from build123d import *

# Parameters (mm, degrees)
SKETCH1_W               = 127
SKETCH1_H               = 127
BOSS_EXTRUDE1_DEPTH     = 6.35
BOSS_EXTRUDE2_DEPTH     = 6.35
BOSS_EXTRUDE3_DEPTH     = 6.35
SKETCH6_W               = 127
SKETCH6_H               = 25.4
BOSS_EXTRUDE4_DEPTH     = 8.89
SKETCH7_R               = 8.1915
CUT_EXTRUDE1_DEPTH      = 8.89
SKETCH8_W               = 109.22
SKETCH8_H               = 25.4
BOSS_EXTRUDE5_DEPTH     = 8.89
SKETCH9_W               = 12.7
SKETCH9_H               = 12.7
BOSS_EXTRUDE6_DEPTH     = 29.21
SKETCH10_W              = 12.7
SKETCH10_H              = 12.7
BOSS_EXTRUDE7_DEPTH     = 31.75
MIRROR5_COPY_1_SKETCH_W = 12.7
MIRROR5_COPY_1_SKETCH_H = 12.7
MIRROR5_COPY_1_DEPTH    = 29.21
MIRROR5_COPY_2_SKETCH_W = 12.7
MIRROR5_COPY_2_SKETCH_H = 12.7
MIRROR5_COPY_2_DEPTH    = 31.75
FILLET1_R               = 2.54
SKETCH11_W              = 29.21
SKETCH11_H              = 19.05
CUT_EXTRUDE2_DEPTH      = 6.35
SKETCH12_R              = 12.7
SKETCH12_R_2            = 8.1915
BOSS_EXTRUDE8_DEPTH     = 6.35
SKETCH13_R              = 2.1
CUT_EXTRUDE3_DEPTH      = 12.7
MIRROR8_COPY_1_SKETCH_R = 2.1
MIRROR8_COPY_1_DEPTH    = 12.7
SKETCH14_R              = 2.1
CUT_EXTRUDE4_DEPTH      = 25.4
SKETCH15_W              = 8.89
SKETCH15_H              = 44.45
CUT_EXTRUDE5_DEPTH      = 6.35
SKETCH16_W              = 12.7
SKETCH16_H              = 2.54
CUT_EXTRUDE6_DEPTH      = 6.35
CUT_EXTRUDE7_REACH      = 173.586
SKETCH18_W              = 50.530596201
SKETCH18_H              = 73.67869055
SKETCH19_W              = 46.387649415
SKETCH19_H              = 80.970556506
CUT_EXTRUDE8_DEPTH      = 29.21


with BuildPart() as part:
    # Sketch1 → Boss-Extrude1 (new body)
    with BuildSketch(Plane(origin=(0, 0, 0), x_dir=(1, 0, 0), z_dir=(0, 1, 0))):
        Rectangle(SKETCH1_W, SKETCH1_H)
    extrude(amount=BOSS_EXTRUDE1_DEPTH)

    # Sketch3 → Boss-Extrude2 (add, symmetric)
    with BuildSketch(Plane(origin=(31.75, 0, 0), x_dir=(0, 0, -1), z_dir=(1, 0, 0))):
        with BuildLine():
            Line((-43.434, 6.35), (-3.175, 6.35))
            Line((-3.175, 6.35), (-3.175, 19.05))
            Line((-3.175, 19.05), (-12.065, 19.05))
            ThreePointArc((-12.065, 19.05), (-23.3045, 7.8105), (-34.544, 19.05))
            Line((-34.544, 19.05), (-43.434, 19.05))
            Line((-43.434, 19.05), (-43.434, 6.35))
        make_face()
    boss_extrude2 = extrude(amount=BOSS_EXTRUDE2_DEPTH, both=True)

    # Sketch5 → Boss-Extrude3 (add, symmetric)
    with BuildSketch(Plane(origin=(-31.75, 0, 0), x_dir=(0, 0, -1), z_dir=(1, 0, 0))):
        with BuildLine():
            Line((-43.434, 6.35), (-3.175, 6.35))
            Line((-3.175, 6.35), (-3.175, 19.05))
            Line((-3.175, 19.05), (-12.065, 19.05))
            ThreePointArc((-12.065, 19.05), (-23.3045, 7.8105), (-34.544, 19.05))
            Line((-34.544, 19.05), (-43.434, 19.05))
            Line((-43.434, 19.05), (-43.434, 6.35))
        make_face()
    boss_extrude3 = extrude(amount=BOSS_EXTRUDE3_DEPTH, both=True)

    # Mirror1: Boss-Extrude2, Boss-Extrude3 across plane
    add(boss_extrude2.mirror(Plane.XY))
    add(boss_extrude3.mirror(Plane.XY))

    # Sketch6 → Boss-Extrude4 (add)
    with BuildSketch(Plane(origin=(63.5, 0, 0), x_dir=(0, 0, -1), z_dir=(1, 0, 0))):
        with Locations((0, 19.05)):
            Rectangle(SKETCH6_W, SKETCH6_H)
    boss_extrude4 = extrude(amount=-BOSS_EXTRUDE4_DEPTH)

    # Sketch7 → Cut-Extrude1 (cut)
    with BuildSketch(Plane.ZY.offset(-54.61)):
        with Locations((0, 19.05)):
            Circle(SKETCH7_R)
    cut_extrude1 = extrude(amount=-CUT_EXTRUDE1_DEPTH, mode=Mode.SUBTRACT)

    # Mirror2: Boss-Extrude4, Cut-Extrude1 across plane
    add(boss_extrude4.mirror(Plane(origin=(0, 0, 0), x_dir=(0, 0, 1), z_dir=(1, 0, 0))))
    add(cut_extrude1.mirror(Plane(origin=(0, 0, 0), x_dir=(0, 0, 1), z_dir=(1, 0, 0))), mode=Mode.SUBTRACT)

    # Sketch8 → Boss-Extrude5 (add)
    with BuildSketch(Plane(origin=(0, 0, -63.5), x_dir=(-1, 0, 0), z_dir=(0, 0, -1))):
        with Locations((0, 19.05)):
            Rectangle(SKETCH8_W, SKETCH8_H)
    boss_extrude5 = extrude(amount=-BOSS_EXTRUDE5_DEPTH)

    # Mirror3: Boss-Extrude5 across plane
    add(boss_extrude5.mirror(Plane.XY))

    # Sketch9 → Boss-Extrude6 (add)
    with BuildSketch(Plane(origin=(63.5, 0, 0), x_dir=(0, 0, -1), z_dir=(1, 0, 0))):
        with Locations((57.15, 25.4)):
            Rectangle(SKETCH9_W, SKETCH9_H)
    boss_extrude6 = extrude(amount=BOSS_EXTRUDE6_DEPTH)

    # Sketch10 → Boss-Extrude7 (add)
    with BuildSketch(Plane.XZ.offset(-19.05)):
        with Locations((86.36, -57.15)):
            Rectangle(SKETCH10_W, SKETCH10_H)
    boss_extrude7 = extrude(amount=BOSS_EXTRUDE7_DEPTH)

    # Mirror4: Boss-Extrude6, Boss-Extrude7 across plane
    add(boss_extrude6.mirror(Plane.XY))
    add(boss_extrude7.mirror(Plane.XY))

    # Mirror5: Boss-Extrude6, Boss-Extrude7 across plane
    add(boss_extrude6.mirror(Plane(origin=(0, 0, 0), x_dir=(0, 0, 1), z_dir=(1, 0, 0))))
    add(boss_extrude7.mirror(Plane(origin=(0, 0, 0), x_dir=(0, 0, 1), z_dir=(1, 0, 0))))

    # Mirror5 copy 1 sketch → Mirror5 copy 1 (add)
    with BuildSketch(Plane.ZY.offset(63.5)):
        with Locations((57.15, 25.4)):
            Rectangle(MIRROR5_COPY_1_SKETCH_W, MIRROR5_COPY_1_SKETCH_H)
    extrude(amount=MIRROR5_COPY_1_DEPTH)

    # Mirror5 copy 2 sketch → Mirror5 copy 2 (add)
    with BuildSketch(Plane(origin=(0, 19.05, 0), x_dir=(-1, 0, 0), z_dir=(0, -1, 0))):
        with Locations((86.36, -57.15)):
            Rectangle(MIRROR5_COPY_2_SKETCH_W, MIRROR5_COPY_2_SKETCH_H)
    extrude(amount=MIRROR5_COPY_2_DEPTH)

    # Fillet1
    fillet1_edges = [part.edges().sort_by_distance(p)[0] for p in [
        (92.71, 9.525, -63.5),
        (92.71, 9.525, -50.8),
        (71.755, 19.05, -63.5),
        (71.755, 19.05, -50.8),
        (80.01, 19.05, -57.15),
        (80.01, 3.175, -50.8),
        (80.01, 3.175, -63.5),
        (92.71, -12.7, -57.15),
        (86.36, -12.7, -50.8),
        (80.01, -12.7, -57.15),
        (86.36, -12.7, -63.5),
        (92.71, 9.525, 63.5),
        (92.71, 9.525, 50.8),
        (71.755, 19.05, 50.8),
        (71.755, 19.05, 63.5),
        (92.71, -12.7, 57.15),
        (86.36, -12.7, 63.5),
        (80.01, -12.7, 57.15),
        (80.01, 3.175, 63.5),
        (86.36, -12.7, 50.8),
        (80.01, 3.175, 50.8),
        (80.01, 19.05, 57.15),
        (-92.71, 9.525, -63.5),
        (-92.71, 9.525, -50.8),
        (-71.755, 19.05, -50.8),
        (-71.755, 19.05, -63.5),
        (-92.71, -12.7, -57.15),
        (-86.36, -12.7, -63.5),
        (-80.01, -12.7, -57.15),
        (-80.01, 3.175, -63.5),
        (-86.36, -12.7, -50.8),
        (-80.01, 3.175, -50.8),
        (-80.01, 19.05, -57.15),
        (-92.71, 9.525, 63.5),
        (-92.71, 9.525, 50.8),
        (-71.755, 19.05, 63.5),
        (-71.755, 19.05, 50.8),
        (-80.01, 19.05, 57.15),
        (-80.01, 3.175, 50.8),
        (-80.01, 3.175, 63.5),
        (-92.71, -12.7, 57.15),
        (-86.36, -12.7, 50.8),
        (-80.01, -12.7, 57.15),
        (-86.36, -12.7, 63.5),
    ]]
    fillet(fillet1_edges, radius=FILLET1_R)

    # Sketch11 → Cut-Extrude2 (cut)
    with BuildSketch(Plane(origin=(0, 6.35, 0), x_dir=(1, 0, 0), z_dir=(0, 1, 0))):
        with Locations((6.985, 0)):
            Rectangle(SKETCH11_W, SKETCH11_H)
    extrude(amount=-CUT_EXTRUDE2_DEPTH, mode=Mode.SUBTRACT)

    # Sketch12 → Boss-Extrude8 (add)
    with BuildSketch(Plane(origin=(63.5, 0, 0), x_dir=(0, 0, -1), z_dir=(1, 0, 0))):
        with Locations(Location((0, 19.05, 0), (0, 0, 90))):
            Circle(SKETCH12_R)
        with Locations(Location((0, 19.05, 0), (0, 0, 180))):
            Circle(SKETCH12_R_2, mode=Mode.SUBTRACT)
    boss_extrude8 = extrude(amount=BOSS_EXTRUDE8_DEPTH)

    # Mirror6: Boss-Extrude8 across plane
    add(boss_extrude8.mirror(Plane(origin=(0, 0, 0), x_dir=(0, 0, 1), z_dir=(1, 0, 0))))

    # Sketch13 → Cut-Extrude3 (cut)
    with BuildSketch(Plane(origin=(0, 19.05, 0), x_dir=(1, 0, 0), z_dir=(0, 1, 0))):
        with Locations(Location((31.75, -38.989, 0), (0, 0, 270))):
            Circle(SKETCH13_R)
        with Locations(Location((31.75, -7.62, 0), (0, 0, 270))):
            Circle(SKETCH13_R)
    cut_extrude3 = extrude(amount=-CUT_EXTRUDE3_DEPTH, mode=Mode.SUBTRACT)

    # Mirror7: Cut-Extrude3 across plane
    add(cut_extrude3.mirror(Plane.XY), mode=Mode.SUBTRACT)

    # Mirror8: Cut-Extrude3 across plane
    add(cut_extrude3.mirror(Plane(origin=(0, 0, 0), x_dir=(0, 0, 1), z_dir=(1, 0, 0))), mode=Mode.SUBTRACT)

    # Mirror8 copy 1 sketch → Mirror8 copy 1 (cut)
    with BuildSketch(Plane(origin=(0, 19.05, 0), x_dir=(-1, 0, 0), z_dir=(0, 1, 0))):
        with Locations(Location((31.75, -38.989, 0), (0, 0, 270))):
            Circle(MIRROR8_COPY_1_SKETCH_R)
        with Locations(Location((31.75, -7.62, 0), (0, 0, 270))):
            Circle(MIRROR8_COPY_1_SKETCH_R)
    extrude(amount=-MIRROR8_COPY_1_DEPTH, mode=Mode.SUBTRACT)

    # Sketch14 → Cut-Extrude4 (cut)
    with BuildSketch(Plane(origin=(0, 31.75, 0), x_dir=(1, 0, 0), z_dir=(0, 1, 0))):
        with Locations(Location((-58.71, 58.71, 0), (0, 0, 270))):
            Circle(SKETCH14_R)
        with Locations(Location((58.71, -58.71, 0), (0, 0, 270))):
            Circle(SKETCH14_R)
    extrude(amount=-CUT_EXTRUDE4_DEPTH, mode=Mode.SUBTRACT)

    # Sketch15 → Cut-Extrude5 (cut)
    with BuildSketch(Plane(origin=(0, 6.35, 0), x_dir=(1, 0, 0), z_dir=(0, 1, 0))):
        with Locations((49.165, 0)):
            Rectangle(SKETCH15_W, SKETCH15_H)
    cut_extrude5 = extrude(amount=-CUT_EXTRUDE5_DEPTH, mode=Mode.SUBTRACT)

    # Mirror9: Cut-Extrude5 across plane
    add(cut_extrude5.mirror(Plane(origin=(0, 0, 0), x_dir=(0, 0, 1), z_dir=(1, 0, 0))), mode=Mode.SUBTRACT)

    # Sketch16 → Cut-Extrude6 (cut)
    with BuildSketch(Plane(origin=(0, 6.35, 0), x_dir=(1, 0, 0), z_dir=(0, 1, 0))):
        with Locations((-27.94, -1.27)):
            Rectangle(SKETCH16_W, SKETCH16_H)
    extrude(amount=-CUT_EXTRUDE6_DEPTH, mode=Mode.SUBTRACT)

    # Sketch18 → Cut-Extrude7 (cut, up to next)
    with BuildSketch(Plane.ZY.offset(63.5), mode=Mode.PRIVATE) as cut_extrude7_sk1:
        with Locations((60.834321125, 15.733047456)):
            Rectangle(SKETCH18_W, SKETCH18_H)
    cut_extrude7_tool1 = extrude(cut_extrude7_sk1.sketch, amount=CUT_EXTRUDE7_REACH, mode=Mode.PRIVATE) & part.part
    add(cut_extrude7_tool1.solids().sort_by_distance((-63.5, 15.733047, 60.834321))[0], mode=Mode.SUBTRACT)

    # Sketch19 → Cut-Extrude8 (cut)
    with BuildSketch(Plane(origin=(63.5, 0, 0), x_dir=(0, 0, -1), z_dir=(1, 0, 0))):
        with Locations((60.941888133, 13.904143716)):
            Rectangle(SKETCH19_W, SKETCH19_H)
    extrude(amount=CUT_EXTRUDE8_DEPTH, mode=Mode.SUBTRACT)


solid = part.part
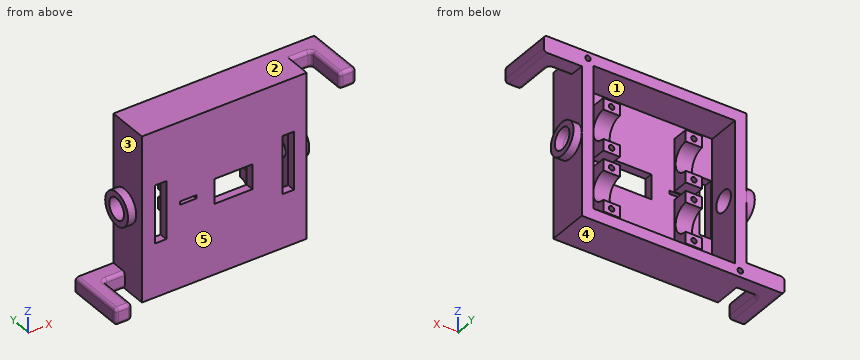
Work out the finished part from the listing and answer in its coordinate system (mm). Face numbers are marked on the shaded views. A direction names the side the tool comes from. Coordinates: 2 decimals unless noted, no trailing zeros. Write each loop counter-clockwise with the first axis right and the second up, starting at its lowest first coordinate (ties: lowest second). Pieces come first, ordered by that corner, then holes. Notation, with made-up numbers: M -29.75,70 L -3.75,70 A37 ccw -3.75,108 Z; hole C -33,13 d10. An arc over 180 degrees is marked long. Use one line per item in the form item = value. Start each with the question number.
1. The mould has two halves that part along Z. Classify the marked faces 3, 4 and 5: released by +Z, released by -Z, zero draft, split by the parting line, or undercut.
2. A tool of negligible diameter and unlimited length cuts with its end or side. For the marked faces 1 and 2, from which of +Z, -Z, +X, -X, +Y, -Y can it reach the whole face along a straight path? Write none if from no direction.
3. Each of these flat-tipped pins is pushed along its axis until it touches: P1, Ø4.5, axis at x = 33.5, z = -6.5, coming from the +Y side; P2, Ø2, axis at x = -59, z = -58, coming from the +Y side; P3, Ø3, axis at x = 52, z = -48.5, coming from the -Y side; P4, Ø5.5, axis at x = 58.71, z = 58.71, coming from the +Y side. Where does it stop, or does it pass through?
4. The part is cut by section B-B (y = -2). Give the vertices of the cut face in (x, z).
5. The part is cut by section D-D (x = -40). Give the vertices of the cut face in (y, z), plus the area to 3 significant figures.
6. The part is cut by section C-C (z = 58.71). Give the vertices of the cut face in (x, y).
7. The part is cut by section A-A (x = 58.71). Give the vertices of the cut face in (y, z), plus the area to 3 significant figures.
8. Straight lines are drawn through the part: probe 1 along X at (y, z) = (11.5, -43); probe 2 along Z at (x, y) = (59, 19); probe 3 along Z at (x, y) = (48, 11). For each, find the intervals that lie inside material, in ascending order. Write a range as from..to.
Evaluation:
q1.face_3 = undercut
q1.face_4 = released by -Z
q1.face_5 = zero draft
q2.face_1 = +Y
q2.face_2 = +Z, +X, -X, +Y, -Y
q3.P1 = 19.05
q3.P2 = 6.35
q3.P3 = 0
q3.P4 = 31.75
q4.outline = M -92.71,-60.96 A2.54 ccw -90.17,-63.5 L -82.55,-63.5 A2.54 ccw -80.01,-60.96 L -80.01,-53.34 A2.54 ccw -82.55,-50.8 L -90.17,-50.8 A2.54 ccw -92.71,-53.34 Z; M 80.01,53.34 A2.54 ccw 82.55,50.8 L 90.17,50.8 A2.54 ccw 92.71,53.34 L 92.71,60.96 A2.54 ccw 90.17,63.5 L 82.55,63.5 A2.54 ccw 80.01,60.96 Z
q5.outline = M 0,-63.5 L 31.75,-63.5 L 31.75,-54.61 L 6.35,-54.61 L 6.35,54.61 L 31.75,54.61 L 31.75,63.5 L 0,63.5 Z
q5.area = 1,260 mm^2
q6.outline = M -63.5,0 L 63.5,0 L 63.5,19.05 L 77.47,19.05 A2.54 cw 80.01,16.51 L 80.01,-10.16 A2.54 ccw 82.55,-12.7 L 90.17,-12.7 A2.54 ccw 92.71,-10.16 L 92.71,31.75 L 60.81,31.75 L 60.81,6.35 L 56.61,6.35 L 56.61,31.75 L -63.5,31.75 Z
q7.outline = M 0,-63.5 L 31.75,-63.5 L 31.75,56.61 L 6.35,56.61 L 6.35,60.81 L 31.75,60.81 L 31.75,63.5 L 0,63.5 Z; hole C 19.05,0 d16.38
q7.area = 3,710 mm^2
q8.probe_1 = -63.5..-54.61, -38.1..-25.4, 25.4..38.1, 54.61..63.5
q8.probe_2 = -63.5..-8.19, 8.19..56.63, 60.79..63.5
q8.probe_3 = -63.5..-54.61, 54.61..63.5
